Model file for the job. Use its own axes, mm. Face numbers are marked on the shaded views. A direction names the side the tool comes from. Round coordinates to 2 decimals unless told otherwise and drop trailing zeros. Order: outer loops, then holes, each group sorted by start corner. A loop starts at its lowest first (then second) coordinate and runs counter-clockwise, first axis right, second up. Notation, with made-up numbers: (-12.75, 31.5) -> (1.25, 31.5) arc R22 ccw to (1.25, 64.5) -> close; hole circle Ø1 at (-27.5, 88). An arc over 180 degrees is marked (long way). Put each result on its own line as item: value. Start each with the question number.
Q1. 3-axis set-ups, long thin cutter, end or side, ignore diameter. For the marked faces 4 and 5: which of +Z, -Z, +X, -X, +Y, -Y reach the whole face in a straight line?
Q2. Cut at B-B, the plane y = -6. List the corners of the cut face in (x, z).
Q3. Pull direction Z, two halves, no side cores. Call the marked faces 1, 2 and 3: released by +Z, released by -Z, zero draft, split by the parting line, or undercut.
Q4. Cut at A-A, the plane z = 0. List the corners of the cut face in (x, y).
Q5. Probe L1, parallel to X at y = -5, z = 0; L2, parallel to X at y = -5.25, z = -3; L3, parallel to Z at x = -6, y = -8.75. List the from-to ranges inside material, lowest first.
Q6. Flat gauge pins, fed straight in: P1, Ø1.7, axis at y = -4, z = -13, coming from the -X side; P2, Ø2.5, axis at y = -7, z = -12.5, coming from the +X side; P3, Ø5, axis at x = 4.5, z = 14.5, coming from the -Y side. Where does each tip first touch, or does it go through?
from build123d import *

# Parameters (mm, degrees)
F1_DEPTH     = 10
F2_R         = 5
F3_R         = 5
F4_R         = 5
F5_R         = 5
F6_R         = 5
F7_T1_DEPTH  = 12.9209860369
F7_T3_DEPTH  = 12.9209860369
F7_T5_DEPTH  = 5.6410319467
F7_T8_ANGLE  = 41.3143422779
F7_T10_ANGLE = 104.5599421702
F7_T12_ANGLE = 42.0246275794
F7_T14_ANGLE = 41.3143422779
F7_T16_ANGLE = 104.5599421702
F7_T18_ANGLE = 42.0246275794
F8_T1_DEPTH  = 12.9209860369
F8_T3_DEPTH  = 12.9209860369
F8_T5_DEPTH  = 5.6410319467
F8_T8_ANGLE  = 42.0246275794
F8_T10_ANGLE = 42.0246275794
F8_T12_ANGLE = 104.5599421702
F8_T14_ANGLE = 104.5599421702
F8_T16_ANGLE = 41.3143422779
F8_T18_ANGLE = 41.3143422779


# Not quite as in the source:
# - a fillet or chamfer that OpenCascade refuses, or shapes differently, is made with other operations: its cross-section is extruded or revolved along the edge and cut away or added


with BuildPart() as f1:
    # F0 (on Front) → F1 (new body)
    with BuildSketch(Plane.XZ):
        with BuildLine():
            ThreePointArc((-5, -8.6602540378), (0, 10), (5, -8.6602540378))
            Line((5, -8.6602540378), (6.25, -10.8253175473))
            Line((6.25, -10.8253175473), (8, -13.8564064606))
            Line((8, -13.8564064606), (8, -9.6046863561))
            ThreePointArc((8, -9.6046863561), (12.3033115605, 2.2087382474), (4.1595701998, 11.7876195965))
            ThreePointArc((4.1595701998, 11.7876195965), (0, 12.5), (-4.1595701998, 11.7876195965))
            ThreePointArc((-4.1595701998, 11.7876195965), (-12.3033115605, 2.2087382474), (-8, -9.6046863561))
            Line((-8, -9.6046863561), (-8, -13.8564064606))
            Line((-8, -13.8564064606), (-6.25, -10.8253175473))
            Line((-6.25, -10.8253175473), (-5, -8.6602540378))
        make_face()
        with BuildLine():
            ThreePointArc((-4.1595701998, 11.7876195965), (0, 12.5), (4.1595701998, 11.7876195965))
            Line((4.1595701998, 11.7876195965), (0, 22.5))
            Line((0, 22.5), (-4.1595701998, 11.7876195965))
        make_face()
    extrude(amount=F1_DEPTH)

    # F2
    f2_edges = [f1.edges().sort_by_distance(p)[0] for p in [
        (-4.15957, -5, 11.78762),
    ]]
    fillet(f2_edges, radius=F2_R)

    # F3
    f3_edges = [f1.edges().sort_by_distance(p)[0] for p in [
        (4.15957, -5, 11.78762),
    ]]
    fillet(f3_edges, radius=F3_R)

    # F4
    f4_edges = [f1.edges().sort_by_distance(p)[0] for p in [
        (-5, -5, -8.660254),
    ]]
    fillet(f4_edges, radius=F4_R)

    # F5
    f5_edges = [f1.edges().sort_by_distance(p)[0] for p in [
        (-8, -5, -9.604686),
    ]]
    fillet(f5_edges, radius=F5_R)

    # F6
    f6_edges = [f1.edges().sort_by_distance(p)[0] for p in [
        (8, -5, -9.604686),
        (5, -5, -8.660254),
    ]]
    fillet(f6_edges, radius=F6_R)

    # F7: fillet of radius 1.4 on 2 edges, made by hand

    # F7_s2 → F7_t1 (cut)
    with BuildSketch(Plane(origin=(-4.1819067631, 0, 10.7699050398), x_dir=(0, 1, 0), z_dir=(-0.3619658098, 0, 0.9321913712))):
        with BuildLine():
            ThreePointArc((-8.6, -8.1442307215), (-9.5899494937, -7.7341802151), (-10, -6.7442307215))
            Line((-10, -6.7442307215), (-10, -8.1442307215))
            Line((-10, -8.1442307215), (-8.6, -8.1442307215))
        make_face()
    extrude(amount=F7_T1_DEPTH, mode=Mode.SUBTRACT)

    # F7_s4 → F7_t3 (cut)
    with BuildSketch(Plane(origin=(8.8588619379, 0, 22.8147367305), x_dir=(0, 1, 0), z_dir=(-0.3619658098, 0, -0.9321913712))):
        with BuildLine():
            ThreePointArc((-8.6, -8.1442307215), (-9.5899494937, -7.7341802151), (-10, -6.7442307215))
            Line((-10, -6.7442307215), (-10, -8.1442307215))
            Line((-10, -8.1442307215), (-8.6, -8.1442307215))
        make_face()
    extrude(amount=F7_T3_DEPTH, mode=Mode.SUBTRACT)

    # F7_s6 → F7_t5 (cut)
    with BuildSketch(Plane.XY.offset(-17.3564064606)):
        with BuildLine():
            ThreePointArc((-8, -8.6), (-7.5899494937, -9.5899494937), (-6.6, -10))
            Line((-6.6, -10), (-8, -10))
            Line((-8, -10), (-8, -8.6))
        make_face()
        with BuildLine():
            ThreePointArc((8, -8.6), (7.5899494937, -9.5899494937), (6.6, -10))
            Line((6.6, -10), (8, -10))
            Line((8, -10), (8, -8.6))
        make_face()
    extrude(amount=F7_T5_DEPTH, mode=Mode.SUBTRACT)

    # F7_s7 → F7_t8 (revolve, cut)
    with BuildSketch(Plane(origin=(4.1819067631, 0, 10.7699050398), x_dir=(0, 1, 0), z_dir=(0.3619658098, 0, 0.9321913712))):
        with BuildLine():
            ThreePointArc((-8.6, 8.1442307215), (-9.5899494937, 7.7341802151), (-10, 6.7442307215))
            Line((-10, 6.7442307215), (-10, 8.1442307215))
            Line((-10, 8.1442307215), (-8.6, 8.1442307215))
        make_face()
    revolve(axis=Axis((-8.0710316963, -10, 15.5276671576), (0, 1, 0)), revolution_arc=F7_T8_ANGLE, mode=Mode.SUBTRACT)

    # F7_s9 → F7_t10 (revolve, cut)
    with BuildSketch(Plane(origin=(0, 0, 0), x_dir=(0, 1, 0), z_dir=(0.8872952661, 0, 0.4612018112))):
        with BuildLine():
            ThreePointArc((-8.6, 12.5), (-9.5899494937, 12.0899494937), (-10, 11.1))
            Line((-10, 11.1), (-10, 12.5))
            Line((-10, 12.5), (-8.6, 12.5))
        make_face()
    revolve(axis=Axis((0, -10, 0), (0, -1, 0)), revolution_arc=F7_T10_ANGLE, mode=Mode.SUBTRACT)

    # F7_s11 → F7_t12 (revolve, cut)
    with BuildSketch(Plane.XY.offset(-11.7153745139)):
        with BuildLine():
            ThreePointArc((-8, -8.6), (-7.5899494937, -9.5899494937), (-6.6, -10))
            Line((-6.6, -10), (-8, -10))
            Line((-8, -10), (-8, -8.6))
        make_face()
    revolve(axis=Axis((-13, -10, -11.7153745139), (0, -1, 0)), revolution_arc=F7_T12_ANGLE, mode=Mode.SUBTRACT)

    # F7_s13 → F7_t14 (revolve, cut)
    with BuildSketch(Plane(origin=(-4.1819067631, 0, 10.7699050398), x_dir=(0, 1, 0), z_dir=(-0.3619658098, 0, 0.9321913712))):
        with BuildLine():
            ThreePointArc((-8.6, -8.1442307215), (-9.5899494937, -7.7341802151), (-10, -6.7442307215))
            Line((-10, -6.7442307215), (-10, -8.1442307215))
            Line((-10, -8.1442307215), (-8.6, -8.1442307215))
        make_face()
    revolve(axis=Axis((8.0710316963, -10, 15.5276671576), (0, -1, 0)), revolution_arc=F7_T14_ANGLE, mode=Mode.SUBTRACT)

    # F7_s15 → F7_t16 (revolve, cut)
    with BuildSketch(Plane(origin=(0, 0, 0), x_dir=(0, 1, 0), z_dir=(-0.6694499722, 0, -0.7428571429))):
        with BuildLine():
            ThreePointArc((-8.6, 12.5), (-9.5899494937, 12.0899494937), (-10, 11.1))
            Line((-10, 11.1), (-10, 12.5))
            Line((-10, 12.5), (-8.6, 12.5))
        make_face()
    revolve(axis=Axis((0, -10, 0), (0, -1, 0)), revolution_arc=F7_T16_ANGLE, mode=Mode.SUBTRACT)

    # F7_s17 → F7_t18 (revolve, cut)
    with BuildSketch(Plane.XY.offset(-11.7153745139)):
        with BuildLine():
            ThreePointArc((8, -8.6), (7.5899494937, -9.5899494937), (6.6, -10))
            Line((6.6, -10), (8, -10))
            Line((8, -10), (8, -8.6))
        make_face()
    revolve(axis=Axis((13, -10, -11.7153745139), (0, 1, 0)), revolution_arc=F7_T18_ANGLE, mode=Mode.SUBTRACT)

    # F8: fillet of radius 1.4 on 8 edges, made by hand

    # F8_s2 → F8_t1 (cut)
    with BuildSketch(Plane(origin=(-4.1819067631, 0, 10.7699050398), x_dir=(0, 1, 0), z_dir=(-0.3619658098, 0, 0.9321913712))):
        with BuildLine():
            ThreePointArc((0, -6.7442307215), (-0.4100505063, -7.7341802151), (-1.4, -8.1442307215))
            Line((-1.4, -8.1442307215), (0, -8.1442307215))
            Line((0, -8.1442307215), (0, -6.7442307215))
        make_face()
    extrude(amount=F8_T1_DEPTH, mode=Mode.SUBTRACT)

    # F8_s4 → F8_t3 (cut)
    with BuildSketch(Plane(origin=(8.8588619379, 0, 22.8147367305), x_dir=(0, 1, 0), z_dir=(-0.3619658098, 0, -0.9321913712))):
        with BuildLine():
            ThreePointArc((0, -6.7442307215), (-0.4100505063, -7.7341802151), (-1.4, -8.1442307215))
            Line((-1.4, -8.1442307215), (0, -8.1442307215))
            Line((0, -8.1442307215), (0, -6.7442307215))
        make_face()
    extrude(amount=F8_T3_DEPTH, mode=Mode.SUBTRACT)

    # F8_s6 → F8_t5 (cut)
    with BuildSketch(Plane.XY.offset(-17.3564064606)):
        with BuildLine():
            ThreePointArc((-6.6, 0), (-7.5899494937, -0.4100505063), (-8, -1.4))
            Line((-8, -1.4), (-8, 0))
            Line((-8, 0), (-6.6, 0))
        make_face()
        with BuildLine():
            ThreePointArc((6.6, 0), (7.5899494937, -0.4100505063), (8, -1.4))
            Line((8, -1.4), (8, 0))
            Line((8, 0), (6.6, 0))
        make_face()
    extrude(amount=F8_T5_DEPTH, mode=Mode.SUBTRACT)

    # F8_s7 → F8_t8 (revolve, cut)
    with BuildSketch(Plane.XY.offset(-11.7153745139)):
        with BuildLine():
            ThreePointArc((6.6, 0), (7.5899494937, -0.4100505063), (8, -1.4))
            Line((8, -1.4), (8, 0))
            Line((8, 0), (6.6, 0))
        make_face()
    revolve(axis=Axis((13, 0, -11.7153745139), (0, 1, 0)), revolution_arc=F8_T8_ANGLE, mode=Mode.SUBTRACT)

    # F8_s9 → F8_t10 (revolve, cut)
    with BuildSketch(Plane.XY.offset(-11.7153745139)):
        with BuildLine():
            ThreePointArc((-6.6, 0), (-7.5899494937, -0.4100505063), (-8, -1.4))
            Line((-8, -1.4), (-8, 0))
            Line((-8, 0), (-6.6, 0))
        make_face()
    revolve(axis=Axis((-13, 0, -11.7153745139), (0, -1, 0)), revolution_arc=F8_T10_ANGLE, mode=Mode.SUBTRACT)

    # F8_s11 → F8_t12 (revolve, cut)
    with BuildSketch(Plane(origin=(0, 0, 0), x_dir=(0, 1, 0), z_dir=(-0.6694499722, 0, -0.7428571429))):
        with BuildLine():
            ThreePointArc((0, 11.1), (-0.4100505063, 12.0899494937), (-1.4, 12.5))
            Line((-1.4, 12.5), (0, 12.5))
            Line((0, 12.5), (0, 11.1))
        make_face()
    revolve(axis=Axis((0, 0, 0), (0, -1, 0)), revolution_arc=F8_T12_ANGLE, mode=Mode.SUBTRACT)

    # F8_s13 → F8_t14 (revolve, cut)
    with BuildSketch(Plane(origin=(0, 0, 0), x_dir=(0, 1, 0), z_dir=(0.8872952661, 0, 0.4612018112))):
        with BuildLine():
            ThreePointArc((0, 11.1), (-0.4100505063, 12.0899494937), (-1.4, 12.5))
            Line((-1.4, 12.5), (0, 12.5))
            Line((0, 12.5), (0, 11.1))
        make_face()
    revolve(axis=Axis((0, 0, 0), (0, -1, 0)), revolution_arc=F8_T14_ANGLE, mode=Mode.SUBTRACT)

    # F8_s15 → F8_t16 (revolve, cut)
    with BuildSketch(Plane(origin=(-4.1819067631, 0, 10.7699050398), x_dir=(0, 1, 0), z_dir=(-0.3619658098, 0, 0.9321913712))):
        with BuildLine():
            ThreePointArc((0, -6.7442307215), (-0.4100505063, -7.7341802151), (-1.4, -8.1442307215))
            Line((-1.4, -8.1442307215), (0, -8.1442307215))
            Line((0, -8.1442307215), (0, -6.7442307215))
        make_face()
    revolve(axis=Axis((8.0710316963, 0, 15.5276671576), (0, -1, 0)), revolution_arc=F8_T16_ANGLE, mode=Mode.SUBTRACT)

    # F8_s17 → F8_t18 (revolve, cut)
    with BuildSketch(Plane(origin=(4.1819067631, 0, 10.7699050398), x_dir=(0, 1, 0), z_dir=(0.3619658098, 0, 0.9321913712))):
        with BuildLine():
            ThreePointArc((0, 6.7442307215), (-0.4100505063, 7.7341802151), (-1.4, 8.1442307215))
            Line((-1.4, 8.1442307215), (0, 8.1442307215))
            Line((0, 8.1442307215), (0, 6.7442307215))
        make_face()
    revolve(axis=Axis((-8.0710316963, 0, 15.5276671576), (0, 1, 0)), revolution_arc=F8_T18_ANGLE, mode=Mode.SUBTRACT)


solid = f1.part
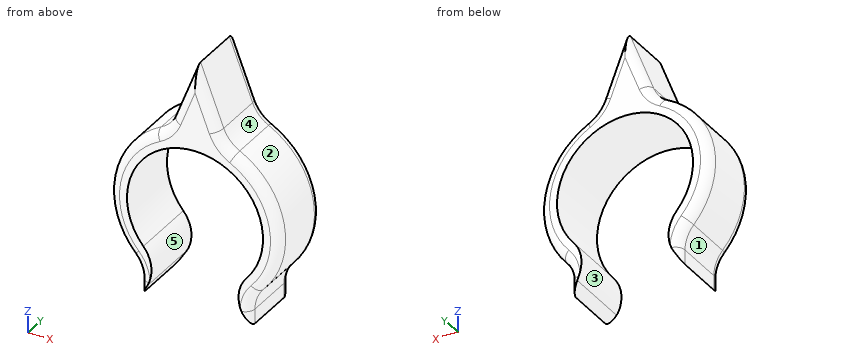
Ans:
1. face 4: +Z, +X, +Y, -Y
1. face 5: +Y, -Y
2. outline: (-9.29, -8.37) arc R5 cw to (-8, -11.72) -> (-8, -13.86) -> (-7.07, -12.25) arc R5 ccw to (-7.6, -6.5) arc R10 cw (long way) to (7.6, -6.5) arc R5 ccw to (7.07, -12.25) -> (8, -13.86) -> (8, -11.72) arc R5 cw to (9.29, -8.37) arc R12.5 ccw to (5.77, 11.09) arc R5 cw to (3.41, 13.72) -> (0, 22.5) -> (-3.41, 13.72) arc R5 cw to (-5.77, 11.09) arc R12.5 ccw to start
3. face 1: released by -Z
3. face 2: split by the parting line
3. face 3: undercut
4. outline: (-12.5, -8.6) arc R1.4 ccw to (-11.1, -10) -> (-10, -10) -> (-10, 0) -> (-11.1, 0) arc R1.4 ccw to (-12.5, -1.4) -> close; (10, -10) -> (11.1, -10) arc R1.4 ccw to (12.5, -8.6) -> (12.5, -1.4) arc R1.4 ccw to (11.1, 0) -> (10, 0) -> close
5. L1: x = -12.5 to -10, 10 to 12.5
5. L2: x = -12.13 to -9.54, 9.54 to 12.13
5. L3: z = 8 to 10.96
6. P1: stops at x = -8
6. P2: stops at x = 8.02
6. P3: stops at y = -9.99
